The listing builds one solid part. Answer for the finished solid, in the listing's coordinates (mm). Face numbers are marked on the shaded views. Give positions to 0.01 mm unless a question says otherwise; leave off trailing zeros. Write each loop counter-clockwise with the first axis right and the second up, starting at its lowest first coordinate (ties: lowest second). Pieces come first, ordered by that corner, then holes.
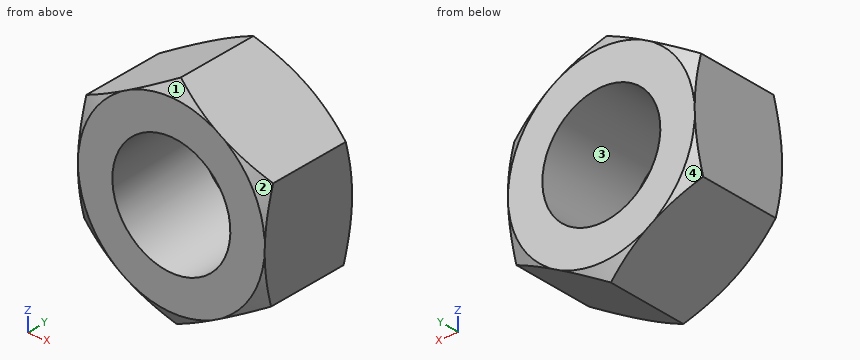
```python
from build123d import *

# Parameters (mm, degrees)
BOSS_EXTRUDE1_DEPTH = 10
SKETCH2_R           = 6
CUT_EXTRUDE1_DEPTH  = 10
SKETCH3_OUTSIDE_W   = 68.948
SKETCH3_OUTSIDE_H   = 71.67
SKETCH3_OUTSIDE_R   = 9.5
CUT_EXTRUDE4_DEPTH  = 12
CUT_EXTRUDE4_DRAFT  = -60
SKETCH4_OUTSIDE_W   = 68.948
SKETCH4_OUTSIDE_H   = 71.67
SKETCH4_OUTSIDE_R   = 9.5
CUT_EXTRUDE5_DEPTH  = 12
CUT_EXTRUDE5_DRAFT  = -60


with BuildPart() as part:
    # Sketch1 → Boss-Extrude1 (new body)
    with BuildSketch(Plane(origin=(0, 0, 0), x_dir=(1, 0, 0), z_dir=(0, 1, 0))):
        Polygon((9.606581004, -5.295935682), (9.389705339, 5.671575352), (-0.216875665, 10.967511034), (-9.606581004, 5.295935682), (-9.389705339, -5.671575352), (0.216875665, -10.967511034), align=None)
    extrude(amount=BOSS_EXTRUDE1_DEPTH)

    # Sketch2 → Cut-Extrude1 (cut)
    with BuildSketch(Plane(origin=(0, 10, 0), x_dir=(1, 0, 0), z_dir=(0, 1, 0))):
        with Locations(Location((0, 0, 0), (0, 0, 270))):
            Circle(SKETCH2_R)
    extrude(amount=-CUT_EXTRUDE1_DEPTH, mode=Mode.SUBTRACT)


with BuildPart() as cut_extrude4_tool:
    # Sketch3 outside → Cut-Extrude4 (with draft: the straight prism first)
    with BuildSketch(Plane(origin=(0, 10, 0), x_dir=(1, 0, 0), z_dir=(0, 1, 0))):
        Rectangle(SKETCH3_OUTSIDE_W, SKETCH3_OUTSIDE_H)
        Circle(SKETCH3_OUTSIDE_R, mode=Mode.SUBTRACT)
    extrude(amount=-CUT_EXTRUDE4_DEPTH)
    # Cut-Extrude4: the draft: its side faces are tilted about the plane it starts from
    cut_extrude4_sides = [cut_extrude4_tool.faces().sort_by_distance(p)[0] for p in [
        (0, 4, 35.835),
        (34.474, 4, 0),
        (0, 4, -35.835),
        (-34.474, 4, 0),
        (-9.5, 4, 0),
    ]]
    draft(cut_extrude4_sides, Plane(origin=(0, 10, 0), x_dir=(1, 0, 0), z_dir=(0, 1, 0)), CUT_EXTRUDE4_DRAFT)


with BuildPart() as part_1:
    add(part.part)

    # Cut-Extrude4: cut by cut_extrude4_tool
    add(cut_extrude4_tool.part, mode=Mode.SUBTRACT)


with BuildPart() as cut_extrude5_tool:
    # Sketch4 outside → Cut-Extrude5 (with draft: the straight prism first)
    with BuildSketch(Plane.XZ):
        Rectangle(SKETCH4_OUTSIDE_W, SKETCH4_OUTSIDE_H)
        Circle(SKETCH4_OUTSIDE_R, mode=Mode.SUBTRACT)
    extrude(amount=-CUT_EXTRUDE5_DEPTH)
    # Cut-Extrude5: the draft: its side faces are tilted about the plane it starts from
    cut_extrude5_sides = [cut_extrude5_tool.faces().sort_by_distance(p)[0] for p in [
        (0, 6, -35.835),
        (34.474, 6, 0),
        (0, 6, 35.835),
        (-34.474, 6, 0),
        (-9.5, 6, 0),
    ]]
    draft(cut_extrude5_sides, Plane.XZ, CUT_EXTRUDE5_DRAFT)


with BuildPart() as part_2:
    add(part_1.part)

    # Cut-Extrude5: cut by cut_extrude5_tool
    add(cut_extrude5_tool.part, mode=Mode.SUBTRACT)


solid = part_2.part
```
Item 1: A cutting plane is placed at A-A, the plane y = 8. Give the vertices of the cut face in (x, z).
Conclusion:
outline: (-9.61, -5.3) - (-0.22, -10.97) - (9.39, -5.67) - (9.61, 5.3) - (0.22, 10.97) - (-9.39, 5.67) - close; hole circle Ø12 at (0, 0)
Item 2: Each of these flat-tipped pins is pushed along its axis until it touches: P1, Ø2, axis at y = 3.5, z = 7.5, coming from the +X side; P2, Ø1.5, axis at y = 7.5, z = -8.5, coming from the +X side; P3, Ø1.5, axis at x = 4.5, y = 4, coming from the +Z side. Where does it stop, or does it pass through?
Conclusion:
P1: stops at x = 7.61
P2: stops at x = 5.62
P3: stops at z = 8.83
Item 3: Determine the mould class of the marked faces 1, 2, 3 and 4 for opening direction X: pulls with the +X half, pulls with the -X half, needs draft (parallel to the pull), parting line crosses it, or undercut.
Conclusion:
face 1: parting line crosses it
face 2: pulls with the +X half
face 3: undercut
face 4: pulls with the -X half
Item 4: Consider probe 1 along X at (y, z) = (3.5, 0); probe 2 along Z at (x, y) = (4.5, 1); probe 3 along X at (y, z) = (3.75, -2.25). Determine where each line is inside the solid, lowest interval first.
Conclusion:
probe 1: x = -9.5 to -6, 6 to 9.5
probe 2: z = -8.37 to -3.97, 3.97 to 8.38
probe 3: x = -9.55 to -5.56, 5.56 to 9.46
